from build123d import *

# Parameters (mm, degrees)
CUT_EXTRUDE1_DEPTH = 9.271
CHAMFER1_SIZE      = 1.16332


with BuildPart() as part:
    # Sketch1 → Revolve2 (revolve)
    with BuildSketch(Plane(origin=(0, 0, 0), x_dir=(1, 0, 0), z_dir=(0, 1, 0))):
        Polygon((0, 14.782898833), (0, -26.212701167), (-6.35, -26.212701167), (-6.35, 2.336898833), (-12.2555, 2.336898833), (-12.2555, 5.511898833), (-11.176, 5.511898833), (-11.176, 14.782898833), align=None)
    revolve(axis=Axis((0, 0, -24.892494163), (0, 0, 1)))

    # Sketch3 → Cut-Extrude1 (cut)
    with BuildSketch(Plane(origin=(0, 0, -14.782898833), x_dir=(-1, 0, 0), z_dir=(0, 0, -1))):
        with BuildLine():
            ThreePointArc((5.334, 9.820968384), (0, 11.176), (-5.334, 9.820968384))
            Line((-5.334, 9.820968384), (5.334, 9.820968384))
        make_face()
        with BuildLine():
            Line((-11.17220811, 0.291104688), (-5.83820811, 9.529863696))
            ThreePointArc((-5.83820811, 9.529863696), (-9.678699913, 5.588), (-11.17220811, 0.291104688))
        make_face()
        with BuildLine():
            Line((-5.83820811, -9.529863696), (-11.17220811, -0.291104688))
            ThreePointArc((-11.17220811, -0.291104688), (-9.678699913, -5.588), (-5.83820811, -9.529863696))
        make_face()
        with BuildLine():
            Line((5.334, -9.820968384), (-5.334, -9.820968384))
            ThreePointArc((-5.334, -9.820968384), (0, -11.176), (5.334, -9.820968384))
        make_face()
        with BuildLine():
            ThreePointArc((5.83820811, -9.529863696), (9.678699913, -5.588), (11.17220811, -0.291104688))
            Line((11.17220811, -0.291104688), (5.83820811, -9.529863696))
        make_face()
        with BuildLine():
            ThreePointArc((11.17220811, 0.291104688), (9.678699913, 5.588), (5.83820811, 9.529863696))
            Line((5.83820811, 9.529863696), (11.17220811, 0.291104688))
        make_face()
    extrude(amount=-CUT_EXTRUDE1_DEPTH, mode=Mode.SUBTRACT)

    # Sketch4 → Cut-Revolve1 (revolve, cut)
    with BuildSketch(Plane(origin=(0, 0, 0), x_dir=(1, 0, 0), z_dir=(0, 1, 0))):
        with BuildLine():
            Line((8.6995, 14.782898833), (11.176, 14.782898833))
            Line((11.176, 14.782898833), (11.176, 13.258898833))
            ThreePointArc((11.176, 13.258898833), (10.119876474, 14.316854353), (8.6995, 14.782898833))
        make_face()
    revolve(axis=Axis((0, 0, -20.186462401), (0, 0, 1)), mode=Mode.SUBTRACT)

    # Chamfer1
    chamfer1_edges = [part.edges().sort_by_distance(p)[0] for p in [
        (6.35, 0, 26.212701167),
    ]]
    chamfer(chamfer1_edges, length=CHAMFER1_SIZE)


solid = part.part
Build history of the part. All positions in model axes, mm. A direction names the side the tool comes from. Coordinates: 2 decimals unless noted, no trailing zeros. Write each loop counter-clockwise with the first axis right and the second up, starting at its lowest first coordinate (ties: lowest second). Pieces come first, ordered by that corner, then holes.
(1) Cut at B-B on z = -4. List the corners of the cut face in (x, y).
(2) Drill centre lines: line 1 (Y direction, x = -0.25, z = 5.5); line 2 (Z direction, x = 7, y = -2.75); line 3 (Z direction, x = 9, y = -6.75). Where is each one in solid material? Low to high.
(3) Pin check, flat tips, straight feed: pin 1 Ø4 at (x, z) = (-6, 2.5) entering from -Y; pin 2 Ø8 at (x, z) = (3, 12.5) entering from -Y; pin 3 Ø12 at (y, z) = (-4, 17) entering from +X. Stop position of each tip, or through.
(4) Cut at C-C on z = 4.5. List the corners of the cut face in (x, y), and give its area (3 significant figures).
(5) 3-axis set-ups, long thin cutter, end or side, ignore diameter. For faces 1 (the flat face through (-8.54, -4.85, -10.06)), 2 (the flat face through (0, 10, -5.512)), 3 (the cylindrical face through (1.38, 6.2, 11.16)), 4 (the flat face through (0, -9.821, -10)): which of +Z, -Z, +X, -X, +Y, -Y reach the whole face in a straight line?
(6) Cut at A-A on x = 0. List the corners of the cut face in (y, z), and give its area (3 significant figures).
Working result:
1. outline: circle Ø24.51 at (0, 0)
2. line 1: y = -6.35 to 6.35
2. line 2: z = -14.78 to -2.34
2. line 3: z = -5.51 to -2.34
3. pin 1: stops at y = -4.93
3. pin 2: stops at y = -6.35
3. pin 3: stops at x = 6.35
4. outline: circle Ø12.7 at (0, 0)
4. area: 127 mm2
5. face 1: -Z, -X, -Y
5. face 2: -Z
5. face 3: +Z
5. face 4: -Z, +X, -X, -Y
6. outline: (-12.26, -5.51) - (-9.82, -5.51) - (-9.82, -14.48) arc R3.22 ccw to (-8.7, -14.78) - (8.7, -14.78) arc R3.22 ccw to (9.82, -14.48) - (9.82, -5.51) - (12.26, -5.51) - (12.26, -2.34) - (6.35, -2.34) - (6.35, 25.05) - (5.19, 26.21) - (-5.19, 26.21) - (-6.35, 25.05) - (-6.35, -2.34) - (-12.26, -2.34) - close
6. area: 621 mm2
